Verification items for the finished model (mm, model axes). A direction names the side the tool comes from. Round coordinates to 2 decimals unless told otherwise and drop trailing zeros. Loops run counter-clockwise (first coordinate to the right, second up) from the corner with the lowest first, then second, coordinate; pieces in that order, holes last. Notation, with made-up numbers: (75.25, -7) -> (92.25, -7) arc R24 ccw to (92.25, 22) -> close; hole circle Ø2 at (43, -9). An arc over 180 degrees is marked (long way). Write item = value, one per line. Start each with the question number.
```python
from build123d import *

# Parameters (mm, degrees)
SKETCH3_W               = 61.087252859
SKETCH3_H               = 56.880141781
SKETCH3_W_2             = 33
SKETCH3_H_2             = 33
CUT_EXTRUDE1_DEPTH      = 22.2
SKETCH6_R               = 2.5
CUT_EXTRUDE5_DEPTH      = 22.2
CUT_EXTRUDE3_REACH      = 35
SKETCH5_R               = 2
G1_8_TAPPED_HOLE1_D     = 8.8
G1_8_TAPPED_HOLE1_DEPTH = 9.356213276
G1_8_TAPPED_HOLE1_TIP   = 2.643786724
CHAMFER1_SIZE           = 0.5


with BuildPart() as part:
    # Sketch2 → Revolve1 (revolve)
    with BuildSketch(Plane.XY):
        Polygon((-3.5, 0), (-22, 0), (-22, 13.2), (-10, 13.2), (-10, 21.2), (-6.35, 21.2), (-6.35, 17.2), (-3.5, 17.2), align=None)
    revolve(axis=Axis((0, 0, 0), (0, 1, 0)))

    # Sketch3 → Cut-Extrude1 (cut, through all)
    with BuildSketch(Plane.XZ):
        with Locations((1.009706659, -0.631066662)):
            Rectangle(SKETCH3_W, SKETCH3_H)
        Rectangle(SKETCH3_W_2, SKETCH3_H_2, mode=Mode.SUBTRACT)
    extrude(amount=-CUT_EXTRUDE1_DEPTH, mode=Mode.SUBTRACT)

    # Sketch6 → Cut-Extrude5 (cut, through all)
    with BuildSketch(Plane.XZ):
        with Locations((-11.525840533, 11.525840533)):
            Circle(SKETCH6_R)
        with Locations((11.525840533, 11.525840533)):
            Circle(SKETCH6_R)
        with Locations((-11.525840533, -11.525840533)):
            Circle(SKETCH6_R)
        with Locations((11.525840533, -11.525840533)):
            Circle(SKETCH6_R)
    extrude(amount=-CUT_EXTRUDE5_DEPTH, mode=Mode.SUBTRACT)

    # Sketch5 → Cut-Extrude3 (cut, up to next)
    with BuildSketch(Plane(origin=(0, 0, -16.5), x_dir=(-1, 0, 0), z_dir=(0, 0, -1)), mode=Mode.PRIVATE) as cut_extrude3_sk1:
        with Locations((0, 6.6)):
            Circle(SKETCH5_R)
    cut_extrude3_tool1 = extrude(cut_extrude3_sk1.sketch, amount=-CUT_EXTRUDE3_REACH, mode=Mode.PRIVATE) & part.part
    add(cut_extrude3_tool1.solids().sort_by_distance((0, 6.6, -16.5))[0], mode=Mode.SUBTRACT)

    # G1/8 Tapped Hole1
    with Locations(Plane(origin=(0, 6.6, -16.5), x_dir=(-1, 0, 0), z_dir=(0, 0, -1))):
        with Locations((0, 0)):
            Hole(G1_8_TAPPED_HOLE1_D / 2, depth=G1_8_TAPPED_HOLE1_DEPTH)
            with Locations((0, 0, -(G1_8_TAPPED_HOLE1_DEPTH + G1_8_TAPPED_HOLE1_TIP / 2))):  # 118° drill point
                Cone(0, G1_8_TAPPED_HOLE1_D / 2, G1_8_TAPPED_HOLE1_TIP, mode=Mode.SUBTRACT)

    # Chamfer1
    chamfer1_edges = [part.edges().sort_by_distance(p)[0] for p in [
        (6.35, 21.2, 0),
        (3.5, 0, 0),
        (-14.025840533, 13.2, -11.525840533),
        (-14.025840533, 0, -11.525840533),
        (9.025840533, 13.2, 11.525840533),
        (9.025840533, 0, 11.525840533),
        (9.025840533, 13.2, -11.525840533),
        (9.025840533, 0, -11.525840533),
        (-14.025840533, 13.2, 11.525840533),
        (-14.025840533, 0, 11.525840533),
        (10, 21.2, 0),
    ]]
    chamfer(chamfer1_edges, length=CHAMFER1_SIZE)


solid = part.part
```
(1) Scan lines: line 1 (X direction, y = 6.75, z = -5.5); line 2 (Z direction, x = 13, y = 6); line 3 (Z direction, x = -11, y = 12.75). Record each from-to range of solid material in increasing order. Write a range as [from, to].
(2) Section check B-B on z = 0. Enter the section's corners in (x, y), then the cut area to 3 significant figures.
(3) Draft check along Y on faces 3 (the cylindrical face through (-1.075, 8.286, -4.307)), 4 (the flat face through (-4, 0, 4)), 5 (the flat face through (-16.5, 7, 0)). Enter one of: +Y half, -Y half, draft (parallel to the pull), parting line (faces both ways), or undercut.
(4) Section check C-C on y = 6.6. Enter the section's corners in (x, z), then the cut area to 3 significant figures.
(5) Section check A-A on x = 0. Give the number of separate pieces and of enclosed holes in the cut face, then the cut area to 3 significant figures.
(6) Access from +Z, -Z, +X, -X, +Y, -Y to the whole of each face (thin tool, end or side, straight path). Record for faces 1 (the flat face through (8, 13.2, 8)), 2 (the conical face through (0.466, 4.501, -5.792)).
(7) Depth check by flat-ended pin: pin 1 Ø6.5 at (x, z) = (-2.5, 2) entering from +Y; pin 2 Ø9 at (x, z) = (0, 0) entering from +Y. Enter the tip coordinate at first touch or a pass-through.
Computed values:
q1.line_1 = [-16.5, -1.99], [1.99, 16.5]
q1.line_2 = [-16.5, -13.54], [-9.51, 9.51], [13.54, 16.5]
q1.line_3 = [-16.5, -14.02], [-9.03, 9.03], [14.02, 16.5]
q2.outline = (-16.5, 0) -> (-4, 0) -> (-3.5, 0.5) -> (-3.5, 17.2) -> (-6.35, 17.2) -> (-6.35, 20.7) -> (-6.85, 21.2) -> (-9.5, 21.2) -> (-10, 20.7) -> (-10, 13.2) -> (-16.5, 13.2) -> close; (3.5, 0.5) -> (4, 0) -> (16.5, 0) -> (16.5, 13.2) -> (10, 13.2) -> (10, 20.7) -> (9.5, 21.2) -> (6.85, 21.2) -> (6.35, 20.7) -> (6.35, 17.2) -> (3.5, 17.2) -> close
q2.area = 424 mm²
q3.face_3 = undercut
q3.face_4 = -Y half
q3.face_5 = draft
q4.outline = (-16.5, -14.55) arc R22 ccw to (-14.55, -16.5) -> (-4.4, -16.5) -> (-4.4, -7.14) -> (-2, -5.7) -> (-2, -2.87) arc R3.5 cw (long way) to (2, -2.87) -> (2, -5.7) -> (4.4, -7.14) -> (4.4, -16.5) -> (14.55, -16.5) arc R22 ccw to (16.5, -14.55) -> (16.5, 14.55) arc R22 ccw to (14.55, 16.5) -> (-14.55, 16.5) arc R22 ccw to (-16.5, 14.55) -> close; hole circle Ø5 at (-11.53, -11.53); hole circle Ø5 at (-11.53, 11.53); hole circle Ø5 at (11.53, -11.53); hole circle Ø5 at (11.53, 11.53)
q4.area = 864 mm²
q5.separate_pieces = 3
q5.enclosed_holes = 0
q5.area = 323 mm²
q6.face_1 = +Y
q6.face_2 = -Z
q7.pin_1 = 20.8
q7.pin_2 = 17.2
